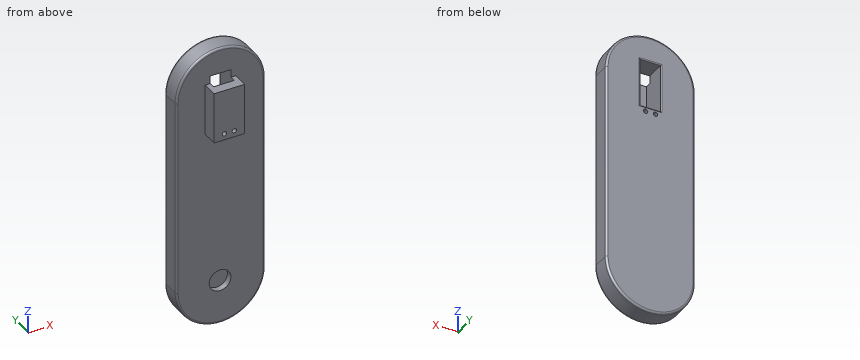
```python
from build123d import *

# Parameters (mm, degrees)
SKETCH1_R           = 2.2
BOSS_EXTRUDE1_DEPTH = 20
FILLET1_R           = 2
SKETCH4_R           = 11
CUT_EXTRUDE2_DEPTH  = 6.35
SKETCH5_W           = 31
SKETCH5_H           = 52
BOSS_EXTRUDE2_DEPTH = 36
SKETCH7_W           = 21
SKETCH7_H           = 49
CUT_EXTRUDE4_DEPTH  = 26
FILLET2_R           = 1
SKETCH8_R           = 2.2
CUT_EXTRUDE5_DEPTH  = 37


with BuildPart() as part:
    # Sketch1 → Boss-Extrude1 (new body)
    with BuildSketch(Plane(origin=(0, 0, 0), x_dir=(1, 0, 0), z_dir=(0, 1, 0))):
        with BuildLine():
            Line((0, 0), (0, 200))
            ThreePointArc((0, 200), (-45, 245), (-90, 200))
            Line((-90, 200), (-90, 0))
            ThreePointArc((-90, 0), (-45, -45), (0, 0))
        make_face()
        with Locations((-50, 34.589613301)):
            Circle(SKETCH1_R, mode=Mode.SUBTRACT)
        with Locations((-40, 34.589613301)):
            Circle(SKETCH1_R, mode=Mode.SUBTRACT)
    extrude(amount=-BOSS_EXTRUDE1_DEPTH)

    # Fillet1
    fillet1_edges = [part.edges().sort_by_distance(p)[0] for p in [
        (-45, -20, -245),
        (-90, -20, -100),
        (-45, -20, 45),
        (-90, 0, -100),
        (-45, 0, -245),
        (0, 0, -100),
        (-45, 0, 45),
        (0, -20, -100),
    ]]
    fillet(fillet1_edges, radius=FILLET1_R)

    # Sketch4 → Cut-Extrude2 (cut)
    with BuildSketch(Plane.XZ.offset(20)):
        with Locations((-45.5, -200)):
            Circle(SKETCH4_R)
    extrude(amount=-CUT_EXTRUDE2_DEPTH, mode=Mode.SUBTRACT)

    # Sketch5 → Boss-Extrude2 (add)
    with BuildSketch(Plane(origin=(0, 0, 0), x_dir=(1, 0, 0), z_dir=(0, 1, 0))):
        with Locations((-45, 15)):
            Rectangle(SKETCH5_W, SKETCH5_H)
    extrude(amount=-BOSS_EXTRUDE2_DEPTH)

    # Sketch7 → Cut-Extrude4 (cut)
    with BuildSketch(Plane(origin=(0, 0, 0), x_dir=(1, 0, 0), z_dir=(0, 1, 0))):
        with Locations((-45, 5.5)):
            Rectangle(SKETCH7_W, SKETCH7_H)
    extrude(amount=-CUT_EXTRUDE4_DEPTH, mode=Mode.SUBTRACT)

    # Fillet2
    fillet2_edges = [part.edges().sort_by_distance(p)[0] for p in [
        (-45, 0, 19),
        (-34.5, 0, -5.5),
        (-45, 0, -30),
        (-55.5, 0, -5.5),
    ]]
    fillet(fillet2_edges, radius=FILLET2_R)

    # Sketch8 → Cut-Extrude5 (cut, through all)
    with BuildSketch(Plane(origin=(0, 0, 0), x_dir=(1, 0, 0), z_dir=(0, 1, 0))):
        with Locations((-50, 34.7)):
            Circle(SKETCH8_R)
        with Locations((-40, 34.7)):
            Circle(SKETCH8_R)
    extrude(amount=-CUT_EXTRUDE5_DEPTH, mode=Mode.SUBTRACT)


solid = part.part
```
For this review, take the finished solid that the model builds, in its own axes (mm). Round coordinates to 2 decimals unless told otherwise and drop trailing zeros. Loops run counter-clockwise (first coordinate to the right, second up) from the corner with the lowest first, then second, coordinate; pieces in that order, holes last.
(1) We need section B-B (x = -45). Give the boundary of the cut face in (y, z), plus the area to 3 significant figures.
Returned:
outline: (-36, -41) - (-20, -41) - (-20, -189.01) - (-13.65, -189.01) - (-13.65, -210.99) - (-20, -210.99) - (-20, -243) arc R2 ccw to (-18, -245) - (-2, -245) arc R2 ccw to (0, -243) - (0, -31) arc R1 ccw to (-1, -30) - (-26, -30) - (-26, 11) - (-36, 11) - close; (-20, 19) - (-1, 19) arc R1 ccw to (0, 20) - (0, 43) arc R2 ccw to (-2, 45) - (-18, 45) arc R2 ccw to (-20, 43) - close
area: 5,260 mm2
(2) Clearance check with flat-ended pins moving along their axes: P1, Ø8, axis at x = -34.5, y = -17.5, coming from the +Z side; P2, Ø5, axis at x = -51, y = -20, coming from the +Z side; P3, Ø3.5, axis at x = -40, z = -34.7, coming from the -Y side; P4, Ø8, axis at x = -49.5, y = -25, coming from the +Z side. State where each tip first meets the part, or that it passes through.
Returned:
P1: stops at z = 44.53
P2: stops at z = 44.79
P3: passes through
P4: stops at z = 11
(3) We need section C-C (y = -30). Give the boundary of the cut face in (x, z), plus the area to 3 significant figures.
Returned:
outline: (-60.5, -41) - (-29.5, -41) - (-29.5, 11) - (-60.5, 11) - close; hole circle Ø4.4 at (-50, -34.7); hole circle Ø4.4 at (-40, -34.7)
area: 1,580 mm2
(4) Wall thickness on line 1 along X through (y, z) = (-14, -34.7); line 2 along X through (y, z) = (-21.5, -34.7); line 3 along X through (y, z) = (-25.5, -17): over which ranges is each line inside the solid? List them lowest first.
Returned:
line 1: x = -90 to -52.2, -47.8 to -42.2, -37.8 to 0
line 2: x = -60.5 to -52.2, -47.8 to -42.2, -37.8 to -29.5
line 3: x = -60.5 to -55.5, -34.5 to -29.5
(5) We need section A-A (z = -184). Give the boundary of the cut face in (x, y).
Returned:
outline: (-90, -18) arc R2 ccw to (-88, -20) - (-2, -20) arc R2 ccw to (0, -18) - (0, -2) arc R2 ccw to (-2, 0) - (-88, 0) arc R2 ccw to (-90, -2) - close
